Autodesk Inventor part; units mm, degrees
ref_plane "YZ Plane" through (0, 0, 0) normal (1, 0, 0) x (0, 1, 0)
ref_plane "XZ Plane" through (0, 0, 0) normal (0, 1, 0) x (-1, 0, 0)
ref_plane "XY Plane" through (0, 0, 0) normal (0, 0, 1) x (1, 0, 0)
sketch "Sketch1" plane through (0, 0, 0) normal (0, 1, 0) x (-1, 0, 0)
  line L0 (0, 0) -> (31, 0)
  line L1 (31, 0) -> (31, -12)
  line L2 (31, -12) -> (0, -12)
  line L3 (0, -12) -> (0, 0)
  line L4 (4, -12) -> (27, -12)
  line L5 (27, -12) -> (27, 0)
  line L6 (27, 0) -> (4, 0)
  line L7 (4, 0) -> (4, -12)
  point P0 (27, 0)
  point P1 (4, 0)
  dimension "d230" = 31
  dimension "d231" = 12
  dimension "d232" = 23
  dimension "d234" = 4
extrude "Extrusion1" add sketch "Sketch1" along normal blind 3 contours L0 L7 L2 L3 | L0 L1 L2 L5
extrude "Extrusion2" add sketch "Sketch1" along normal blind 19 and the other way blind 4 contours L0 L5 L2 L7
sketch "Sketch2" plane through (0, 3, 0) normal (0, 1, 0) x (1, 0, 0)
  line L0 (-27, -10) -> (-37, -10)
  line L1 (-37, -10) -> (-37, 22)
  line L2 (-37, 22) -> (-27, 22)
  line L3 (-27, 22) -> (-27, -10)
  line L4 (-27, 12) -> (-27, 0)
  line L5 (-4, 22) -> (6, 22)
  line L6 (6, 22) -> (6, -10)
  line L7 (6, -10) -> (-4, -10)
  line L8 (-4, -10) -> (-4, 22)
  line L9 (-4, 0) -> (-4, 12)
  point P0 (0, 0)
  point P1 (-27, 6)
  point P2 (-27, 6)
  point P3 (-27, 6)
  point P4 (-4, 6)
  point P5 (-4, 6)
  point P6 (-4, 6)
  dimension "d241" = 10
  dimension "d242" = 32
  dimension "d243" = 10
  dimension "d244" = 32
extrude "Extrusion3" add sketch "Sketch2" along normal blind 2
sketch "Sketch3" plane through (0, 0, 0) normal (0, -1, 0) x (1, 0, 0)
  line L0 (-37, -22) -> (-37, 10)
  line L1 (-27, -12) -> (-27, -22)
  line L2 (-37, 10) -> (-27, 10)
  line L3 (-27, 10) -> (-27, -22)
  line L4 (-27, -22) -> (-37, -22)
  line L5 (-37, -22) -> (-37, 10)
  line L6 (6, -22) -> (-4, -22)
  line L7 (6, 10) -> (6, -22)
  line L8 (-4, -22) -> (6, -22)
  line L9 (6, -22) -> (6, 10)
  line L10 (6, 10) -> (-4, 10)
  line L11 (-4, 10) -> (-4, -22)
  point P0 (0, 0)
extrude "Extrusion4" add sketch "Sketch3" along normal blind 2
sketch "Sketch4" plane through (0, 0, 0) normal (0, 1, 0) x (1, 0, 0)
  line L0 (-4, 22) -> (-4, 12)
  line L1 (6, -10) -> (-4, -10)
  line L2 (-4, 22) -> (6, 22)
  line L3 (-27, 22) -> (-37, 22)
  line L4 (-27, 22) -> (-37, 22)
  line L5 (-37, 22) -> (-37, -10)
  line L6 (-37, -10) -> (-27, -10)
  line L7 (-4, 0) -> (-27, 0)
  line L8 (6, -10) -> (-4, -10)
  line L9 (-4, -10) -> (-4, 0)
  line L10 (-4, 0) -> (6, 0)
  line L11 (6, 0) -> (6, -10)
  line L12 (-27, -10) -> (-37, -10)
  line L13 (-37, -10) -> (-37, 0)
  line L14 (-37, 0) -> (-27, 0)
  line L15 (-27, 0) -> (-27, -10)
  line L16 (-27, 12) -> (-37, 12)
  line L17 (-37, 12) -> (-37, 22)
  line L18 (-37, 22) -> (-27, 22)
  line L19 (-27, 22) -> (-27, 12)
  line L20 (0, 12) -> (-4, 12)
  line L21 (-4, 22) -> (6, 22)
  line L22 (-4, 12) -> (6, 12)
  line L23 (6, 12) -> (6, 22)
  line L24 (6, 22) -> (-4, 22)
  line L25 (-4, 22) -> (-4, 12)
  line L26 (-37, 22) -> (-37, -10)
  line L27 (-37, 22) -> (6, 22)
  line L28 (6, 22) -> (6, 12)
  line L29 (6, 12) -> (-37, 12)
  line L30 (-37, 12) -> (-37, 22)
  line L31 (6, -10) -> (-37, -10)
  line L32 (-37, -10) -> (-37, 0)
  line L33 (-37, 0) -> (6, 0)
  line L34 (6, 0) -> (6, -10)
  point P0 (0, 0)
extrude "Extrusion5" add sketch "Sketch4" along normal blind 3 contours L2 L23 L22 L20 L0 | L14 L15 L6 L5 | L19 L16 L5 L3 | L10 L11 L1 L9
extrude "Extrusion6" add sketch "Sketch4" along normal blind 2
sketch "Sketch5" plane through (0, -4, 0) normal (0, -1, 0) x (1, 0, 0)
  circle A0 centre (-21, -6) radius 6
  line L0 (-4, 0) -> (-27, 0)
  line L1 (-27, 0) -> (-27, -12)
  point P0 (0, 0)
  dimension "d255" = 12
  dimension "d256" = 6
  dimension "d257" = 6
extrude "Extrusion7" add sketch "Sketch5" along normal blind 4 contours A0
sketch "Sketch6" plane through (-21, -8, -6) normal (0, -1, 0) x (1, 0, 0)
  circle A0 centre (0, 0) radius 2.5
  circle A1 centre (0, 0) radius 6
  point P0 (21, 6)
  dimension "d260" = 5
  dimension "d261" = 3.5
extrude "Extrusion8" add sketch "Sketch6" along normal blind 3 contours A0
sketch "Sketch7" plane through (-21, -11, -6) normal (0, -1, 0) x (1, 0, 0)
  line L0 (-6, -6) -> (0, -6)
  line L1 (-6, 6) -> (-6, 0)
  circle A0 centre (0, 0) radius 1
  point P0 (21, 6)
  dimension "d266" = 2
  dimension "d267" = 6
  dimension "d268" = 6
extrude "Extrusion9" cut sketch "Sketch7" against normal blind 6
sketch "Sketch22" plane through (0, 5, 0) normal (0, 1, 0) x (1, 0, 0)
  circle A0 centre (1.5, -4.5) radius 2.5
  circle A1 centre (1.5, 16.5) radius 2.5
  line L0 (-4, 22) -> (-4, 12)
  line L1 (-4, 0) -> (-4, 12)
  line L2 (-27, 0) -> (-27, 6)
  line L3 (-4, 6) -> (-27, 6)
  point P0 (0, 0)
  dimension "d271" = 5
  dimension "d272" = 5
  dimension "d273" = 21
  dimension "d274" = 5.5
extrude "Extrusion26" cut sketch "Sketch22" against normal blind 8
properties part number "Langbektang houder"
Part model, mm, in its own coordinate system. A direction names the side the tool comes from. Give positions to 0.01 mm unless a question says otherwise; leave off trailing zeros. Order: outer loops, then holes, each group sorted by start corner. A loop starts at its lowest first (then second) coordinate and runs counter-clockwise, first axis right, second up. Notation, with made-up numbers: (-24.5, -36.5) - (-7.5, -36.5) arc R34 cw to (-7.5, -3.5) - close; hole circle Ø5 at (42, -14.75). An arc over 180 degrees is marked (long way). Use a Markdown table: item, result.
1) Saw through at B-B on x = 1.5. List the corners of the cut face in (y, z), plus the area to 3 significant figures.
Checked values:
| item | result |
|---|---|
| outline | (-2, -22) - (5, -22) - (5, -19) - (-2, -19) - close; (-2, -14) - (5, -14) - (5, 2) - (-2, 2) - close; (-2, 7) - (5, 7) - (5, 10) - (-2, 10) - close; hole (0, -12) - (3, -12) - (3, 0) - (0, 0) - close |
| area | 118 mm² |
2) Flat gauge pins, fed straight in: P1, Ø2, axis at x = -6, z = -1.5, coming from the -Y side; P2, Ø1.5, axis at x = -22.5, y = -0.5, coming from the -Z side; P3, Ø2, axis at x = -23.5, y = 14.5, coming from the -Z side; P4, Ø1.8, axis at x = -24.5, z = -4, coming from the -Y side. Where does each tip first touch, or does it go through?
Checked values:
| item | result |
|---|---|
| P1 | y = -4 |
| P2 | z = -22 |
| P3 | z = -12 |
| P4 | y = -8 |
3) Two-plate mould, pull along X, no slides. Class faces 4 (the flat face through (6, -1, -6)), 5 (the flat face through (-16, 0, -17)), 6 (the flat face through (3, 1, 0)): +X half, -X half, draft (parallel to the pull), parting line (faces both ways), or undercut.
Checked values:
| item | result |
|---|---|
| face 4 | +X half |
| face 5 | undercut |
| face 6 | draft |
4) Probe L1, parallel to Z at x = 1.5, y = 2.5; L2, parallel to X at y = -0.5, z = -16.5; L3, parallel to Z at x = 1.5, y = -0.25. List the from-to ranges inside material, lowest first. Write a range as from..to.
Checked values:
| item | result |
|---|---|
| L1 | -22..-19, -14..-12, 0..2, 7..10 |
| L2 | -37..-27, -4..-1, 4..6 |
| L3 | -22..-19, -14..2, 7..10 |
5) Saw through at A-A on z = -15. List the corners of the cut face in (x, y).
Checked values:
| item | result |
|---|---|
| outline | (-37, -2) - (-27, -2) - (-27, 0) - (-4, 0) - (-4, -2) - (-0.5, -2) - (-0.5, 5) - (-4, 5) - (-4, 2) - (-27, 2) - (-27, 5) - (-37, 5) - close; (3.5, -2) - (6, -2) - (6, 5) - (3.5, 5) - close |
6) Saw through at D-D on x = -27.5. List the corners of the cut face in (y, z).
Checked values:
| item | result |
|---|---|
| outline | (-2, -22) - (5, -22) - (5, 10) - (-2, 10) - close |
7) Saw through at C-C on z = 0.5. List the corners of the cut face in (x, y).
Checked values:
| item | result |
|---|---|
| outline | (-37, -2) - (-27, -2) - (-27, 0) - (-4, 0) - (-4, -2) - (6, -2) - (6, 5) - (-4, 5) - (-4, 2) - (-27, 2) - (-27, 5) - (-37, 5) - close |
8) 3-axis set-ups, long thin cutter, end or side, ignore diameter. For faces 1 (the flat face through (-4, 3, -17)), 2 (the flat face through (-34, 1, -12)), 3 (the flat face through (-15, -2, 0)): which of +Z, -Z, +X, -X, +Y, -Y reach the whole face in a straight line?
Checked values:
| item | result |
|---|---|
| face 1 | -Z, +Y |
| face 2 | -X |
| face 3 | +Z, -Y |
